Geometry check sheet. Reference: the model listing, model coordinates, mm. A direction names the side the tool comes from. Coordinates: 2 decimals unless noted, no trailing zeros. Write each loop counter-clockwise with the first axis right and the second up, starting at its lowest first coordinate (ties: lowest second). Pieces come first, ordered by that corner, then holes. Notation, with made-up numbers: M 18.5,86.25 L 64.5,86.25 A20 cw 64.5,91.25 Z; hole C 55,79.5 d6. An arc over 180 degrees is marked long. Put each result on its own line as item: value. Start each with the question number.
1) Cross-section at B-B on x = -12.5. Record the cut outline in (y, z).
2) Set-up check for faces 4 (the flat face through (-2, 1, -60.362)), 5 (the flat face through (-23, 1, -40.362)), 6 (the flat face through (-25, 1, -43)): record each of +Z, -Z, +X, -X, +Y, -Y from which the full face is reachable in a straight line by a thin tool's end or side.
3) Gauge pin test, flat ends, axial feed: pin 1 (1 mm diameter, centred on y = 2, z = -10, fed in from +X); pin 2 (6 mm diameter, centred on x = -12.5, z = -17.862, fed in from +Y); pin 3 (1 mm diameter, centred on y = 2, z = -12, fed in from -X). Record the tip position at first contact, or that the pin passes through.
4) Cross-section at D-D on y = 1.85. Count the separate pieces of the cut face and the enclosed holes in it, plus the area to 3 significant figures.
5) Cross-section at A-A on x = -2. Record the cut outline in (y, z), plus the area to 3 significant figures.
6) Scan lines: line 1 along Z through (x, y) = (-12.5, 2.05); line 2 along Z through (x, y) = (-24, 1.1); line 3 along Z through (x, y) = (-11, 1.6). Record each from-to range of solid material in increasing order.
7) Cross-section at C-C on z = -51. Record the cut outline in (x, y).
8) Mould release check, pull along Z, two halves, no side actions. Record for faces 1 (the flat face through (-12, 3, -42)), 2 (the flat face through (-1, 1, -45.362)), 3 (the flat face through (-12, 1, 2.138)): released by +Z, released by -Z, zero draft, split by the parting line, or undercut.
Autodesk Inventor part; units mm, degrees
ref_plane "YZ Plane" through (0, 0, 0) normal (1, 0, 0) x (0, 1, 0)
ref_plane "XZ Plane" through (0, 0, 0) normal (0, 1, 0) x (-1, 0, 0)
ref_plane "XY Plane" through (0, 0, 0) normal (0, 0, 1) x (1, 0, 0)
sketch "Boceto1" plane through (0, 0, 0) normal (0, 1, 0) x (-1, 0, 0)
  line L0 (0, 2.138) -> (25, 2.138)
  line L1 (25, 2.138) -> (25, -87.862)
  line L2 (25, -87.862) -> (0, -87.862)
  line L3 (0, -87.862) -> (0, 2.138)
  line L4 (0, 2.138) -> (25, -87.862) construction
  line L5 (25, 2.138) -> (0, -87.862) construction
  circle A0 centre (12.5, -17.862) radius 3.25
  circle A1 centre (12.1754, -67.8599) radius 3.25
  line L6 (25, -5.362) -> (22, -5.362)
  line L7 (22, -5.362) -> (22, -20.362)
  line L8 (22, -20.362) -> (25, -20.362)
  line L9 (25, -20.362) -> (25, -5.362)
  line L10 (22, -40.362) -> (25, -40.362)
  line L11 (25, -25.362) -> (22, -25.362)
  line L12 (22, -25.362) -> (22, -40.362)
  line L13 (25, -40.362) -> (25, -25.362)
  line L14 (22, -60.362) -> (25, -60.362)
  line L15 (25, -45.362) -> (22, -45.362)
  line L16 (22, -45.362) -> (22, -60.362)
  line L17 (25, -60.362) -> (25, -45.362)
  line L18 (22, -80.362) -> (25, -80.362)
  line L19 (25, -65.362) -> (22, -65.362)
  line L20 (22, -65.362) -> (22, -80.362)
  line L21 (25, -80.362) -> (25, -65.362)
  line L22 (12.5, 2.138) -> (12.5, -87.862) construction
  line L23 (0, -5.362) -> (3, -5.362)
  line L24 (3, -5.362) -> (3, -20.362)
  line L25 (3, -20.362) -> (0, -20.362)
  line L26 (0, -20.362) -> (0, -5.362)
  line L27 (3, -40.362) -> (0, -40.362)
  line L28 (0, -25.362) -> (3, -25.362)
  line L29 (3, -25.362) -> (3, -40.362)
  line L30 (0, -40.362) -> (0, -25.362)
  line L31 (3, -60.362) -> (0, -60.362)
  line L32 (0, -45.362) -> (3, -45.362)
  line L33 (3, -45.362) -> (3, -60.362)
  line L34 (0, -60.362) -> (0, -45.362)
  line L35 (3, -80.362) -> (0, -80.362)
  line L36 (0, -65.362) -> (3, -65.362)
  line L37 (3, -65.362) -> (3, -80.362)
  line L38 (0, -80.362) -> (0, -65.362)
  point P0 (0, 0)
  point P1 (12.5, -50)
  point P2 (12.5, -42.862)
  point P3 (23.5, -5.362)
  point P4 (23.5, -25.362)
  point P5 (23.5, -45.362)
  point P6 (23.5, -65.362)
  point P7 (1.5, -5.362)
  point P8 (1.5, -25.362)
  point P9 (1.5, -45.362)
  point P10 (1.5, -65.362)
  point P11 (0, -5.362)
  point P12 (12.5, -42.862)
  dimension "d3" = 25
  dimension "d4" = 25
  dimension "d5" = 90
  dimension "d6" = 6.5
  dimension "d7" = 6.5
  dimension "d8" = 3
  dimension "d9" = 15
  dimension "d10" = 7.5
  dimension "d13" = 20
  dimension "d20" = 25
extrude "Extrusión1" add sketch "Boceto1" along normal blind 3 contours L0 L1 L6 L7 L8 L11 L12 L10 L15 L16 L14 L19 L20 L18 L2 L3 L35 L37 L36 L31 L33 L32 L27 L29 L28 L25 L24 L23
Answer key:
1. outline: M 0,-87.86 L 3,-87.86 L 3,-71.09 L 0,-71.09 Z; M 0,-64.63 L 3,-64.63 L 3,-21.11 L 0,-21.11 Z; M 0,-14.61 L 3,-14.61 L 3,2.14 L 0,2.14 Z
2. face 4: +X, +Y, -Y
2. face 5: -X, +Y, -Y
2. face 6: +Z, -Z, -X, +Y, -Y
3. pin 1: stops at x = -3
3. pin 2: passes through
3. pin 3: stops at x = -22
4. separate pieces: 1
4. enclosed holes: 2
4. area: 1,820 mm²
5. outline: M 0,-87.86 L 3,-87.86 L 3,-80.36 L 0,-80.36 Z; M 0,-65.36 L 3,-65.36 L 3,-60.36 L 0,-60.36 Z; M 0,-45.36 L 3,-45.36 L 3,-40.36 L 0,-40.36 Z; M 0,-25.36 L 3,-25.36 L 3,-20.36 L 0,-20.36 Z; M 0,-5.36 L 3,-5.36 L 3,2.14 L 0,2.14 Z
5. area: 90.0 mm²
6. line 1: z = -87.86 to -71.09, -64.63 to -21.11, -14.61 to 2.14
6. line 2: z = -87.86 to -80.36, -65.36 to -60.36, -45.36 to -40.36, -25.36 to -20.36, -5.36 to 2.14
6. line 3: z = -87.86 to -70.89, -64.83 to -20.75, -14.98 to 2.14
7. outline: M -22,0 L -3,0 L -3,3 L -22,3 Z
8. face 1: zero draft
8. face 2: undercut
8. face 3: released by +Z
